The model under review builds one solid part; all positions refer to its coordinate system, in mm. Face numbers are marked on the shaded views. A direction names the side the tool comes from. Coordinates: 2 decimals unless noted, no trailing zeros. Write each loop counter-clockwise with the first axis right and the second up, starting at its lowest first coordinate (ties: lowest second). Pieces come first, ordered by that corner, then holes. Notation, with made-up numbers: (49, 69.25) - (58, 69.25) arc R23 ccw to (58, 87.25) - close; hole circle Ø2 at (-30, 11). An arc over 180 degrees is marked (long way). Return JSON: item names as keys, results as strings. Group by question number.
(1) We need section D-D on x = 428. State the section outline as (y, z) points.
(2) We need section A-A on z = 78.5. State the section outline as (x, y) points, then the cut area to 3 significant figures.
(3) Tool access review of the marked faces 1 and 2: name each direction out of +Z, -Z, +X, -X, +Y, -Y from which nothing blocks a thin tool from reaching the whole face with its end or side.
(4) We need section C-C on y = 927. State the section outline as (x, z) points.
(5) For pin 1 Ø25 at (x, z) = (392, 111.5) entering from +Y; pin 2 Ø22.5 at (x, y) = (157.5, 757) entering from +Z, all flat-tipped, find the tip position at first contact; note any pin that passes through.
(6) To check wall thickness, follow L1, parallel to Y at x = 118, z = 78; L2, parallel to Y at x = 399.5, z = 138; L3, parallel to X at y = 904, z = 97.5. State the ranges of each line that lie inside material, in increasing order. Write a range as from..to.
(7) We need section B-B on x = 112. State the section outline as (y, z) points, then the cut area to 3 significant figures.
```python
from build123d import *

# Parameters (mm, degrees)
BOSS_EXTRUDE1_DEPTH = 500
SKETCH2_W           = 100
SKETCH2_H           = 121
SKETCH2_W_2         = 95.3
SKETCH2_H_2         = 10
SKETCH2_W_3         = 82.54
SKETCH2_H_3         = 18.8
SKETCH2_H_4         = 22
SKETCH2_W_4         = 250
SKETCH2_H_5         = 45
CUT_EXTRUDE1_DEPTH  = 268


with BuildPart() as part:
    # Sketch1 → Boss-Extrude1 (new body)
    with BuildSketch(Plane(origin=(0, 0, 0), x_dir=(0, 0, -1), z_dir=(1, 0, 0))):
        Polygon((0, 0), (-190, 0), (-200, 10), (-200, 960), (-160, 1000), (7.526077778, 1000), (7.526077778, 1310), (57.526077778, 1310), (407.526077778, 1310), (407.526077778, 1000), (407.526077778, 970), (407.526077778, 820), (407.526077778, 0), align=None)
    extrude(amount=BOSS_EXTRUDE1_DEPTH)

    # Sketch2 → Cut-Extrude1 (cut)
    with BuildSketch(Plane.XY.offset(200)):
        with Locations((250, 889.5)):
            Rectangle(SKETCH2_W, SKETCH2_H)
        with Locations((100, 889.5)):
            Rectangle(SKETCH2_W_2, SKETCH2_H_2)
        with Locations((406.38, 889.5)):
            Rectangle(SKETCH2_W_3, SKETCH2_H_3)
        with Locations((416.666666667, 758.294000626)):
            Rectangle(SKETCH2_W, SKETCH2_H_4)
        with Locations((166.666666667, 758.294000626)):
            Rectangle(SKETCH2_W_4, SKETCH2_H_5)
    extrude(amount=-CUT_EXTRUDE1_DEPTH, mode=Mode.SUBTRACT)


solid = part.part
```
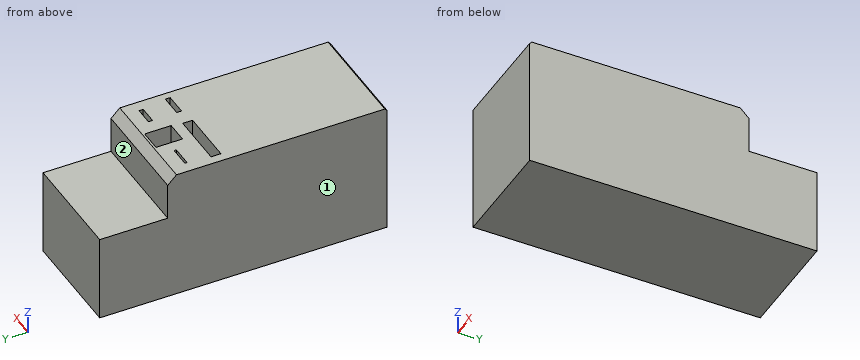
Ans:
{
 "1": {"outline": "(0, -407.53) - (1310, -407.53) - (1310, -7.53) - (1000, -7.53) - (1000, 160) - (960, 200) - (898.9, 200) - (898.9, -68) - (880.1, -68) - (880.1, 200) - (769.29, 200) - (769.29, -68) - (747.29, -68) - (747.29, 200) - (10, 200) - (0, 190) - close"},
 "2": {"outline": "(0, 0) - (500, 0) - (500, 1000) - (0, 1000) - close; hole (41.67, 735.79) - (291.67, 735.79) - (291.67, 780.79) - (41.67, 780.79) - close; hole (52.35, 884.5) - (147.65, 884.5) - (147.65, 894.5) - (52.35, 894.5) - close; hole (200, 829) - (300, 829) - (300, 950) - (200, 950) - close; hole (365.11, 880.1) - (447.65, 880.1) - (447.65, 898.9) - (365.11, 898.9) - close; hole (366.67, 747.29) - (466.67, 747.29) - (466.67, 769.29) - (366.67, 769.29) - close", "area": "472,000 mm²"},
 "3": {"face 1": "+Z, -Z, -X, +Y, -Y", "face 2": "+Z, +X, -X, +Y"},
 "4": {"outline": "(0, -407.53) - (500, -407.53) - (500, 200) - (300, 200) - (300, -68) - (200, -68) - (200, 200) - (0, 200) - close"},
 "5": {"pin 1": "y = 1000", "pin 2": "z = -68"},
 "6": {"L1": "0..735.79, 780.79..884.5, 894.5..1000", "L2": "0..747.29, 769.29..880.1, 898.9..1000", "L3": "0..200, 300..500"},
 "7": {"outline": "(0, -407.53) - (1310, -407.53) - (1310, -7.53) - (1000, -7.53) - (1000, 160) - (960, 200) - (894.5, 200) - (894.5, -68) - (884.5, -68) - (884.5, 200) - (780.79, 200) - (780.79, -68) - (735.79, -68) - (735.79, 200) - (10, 200) - (0, 190) - close", "area": "716,000 mm²"}
}
